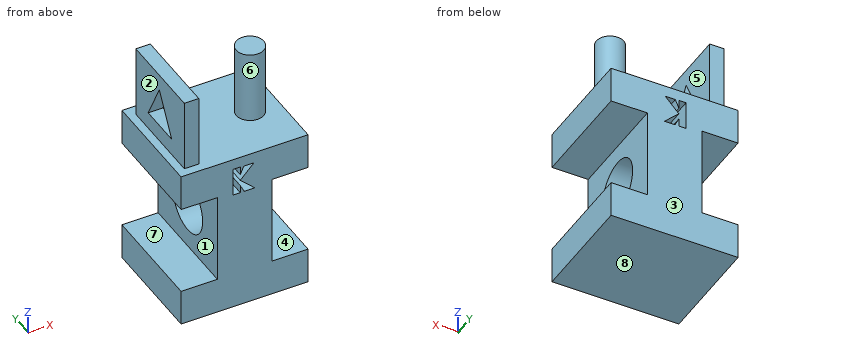
```python
from build123d import *

# Parameters (mm, degrees)
F1_DEPTH  = 76.2
F2_R      = 19.096035609
F3_DEPTH  = 47.498
F4_W      = 10.16
F4_H      = 62.4394440092
F5_DEPTH  = 50.8
F7_DEPTH  = 25.4
F9_DEPTH  = 96.52
F10_R     = 9.6573764136
F11_DEPTH = 50.8


# Not quite as in the source:
# - a feature names something its author has since deleted; it is built from what else it names


with BuildPart() as f1:
    # F0 (on Front) → F1 (new body)
    with BuildSketch(Plane.XZ):
        Polygon((-43.9144560635, -19.0287967878), (-43.9144560635, -44.4287967878), (44.9855439365, -44.4287967878), (44.9855439365, -19.0287967878), (19.5855439365, -19.0287967878), (19.5855439365, 44.4712032122), (44.9855439365, 44.4712032122), (44.9855439365, 69.8712032122), (-43.9144560635, 69.8712032122), (-43.9144560635, 44.4712032122), (-18.5144560635, 44.4712032122), (-18.5144560635, -19.0287967878), align=None)
    extrude(amount=F1_DEPTH)

    # F2 (on face) → F3 (cut)
    with BuildSketch(Plane.YZ.offset(19.5855439365)):
        with Locations((-38.1, 12.7212032122)):
            Circle(F2_R)
    extrude(amount=-F3_DEPTH, mode=Mode.SUBTRACT)

    # F4 (on face) → F5 (join)
    with BuildSketch(Plane.XY.offset(69.8712032122)):
        with Locations((-33.1311938035, -38.6642131489)):
            Rectangle(F4_W, F4_H)
    extrude(amount=F5_DEPTH)

    # F6 (on face) → F7 (cut)
    with BuildSketch(Plane(origin=(-38.2111938035, 0, 0), x_dir=(0, -1, 0), z_dir=(-1, 0, 0))):
        Polygon((53.6283701658, 81.7187428474), (37.7003215253, 109.3182116747), (23.2826862484, 81.7187428474), align=None)
    extrude(amount=-F7_DEPTH, mode=Mode.SUBTRACT)

    # F8 (on face) → F9 (cut)
    with BuildSketch(Plane(origin=(0, 0, 0), x_dir=(-1, 0, 0), z_dir=(0, 1, 0))):
        Polygon((7.511020638, 42.3752516508), (7.511020638, 62.378142029), (2.4668793194, 62.378142029), (2.4668793194, 56.307456918), (0, 62.0944574475), (-7.0838662127, 62.0944574475), (2.4668793194, 51.9569911986), (-7.7034849674, 42.3752516508), (-0.3085337383, 42.3752516508), (2.4668793194, 47.8559471667), (2.4668793194, 42.3752516508), align=None)
    extrude(amount=-F9_DEPTH, mode=Mode.SUBTRACT)

    # F10 (on face) → F11 (join)
    with BuildSketch(Plane.XY.offset(69.8712032122)):
        with Locations((25.0358451158, -38.1)):
            Circle(F10_R)
    extrude(amount=F11_DEPTH)


solid = f1.part
```
Check sheet for the modelled part. Datum: model origin and axes. Units: mm. Face numbers are marked on the shaded views. A direction names the side the tool comes from. Give positions to 0.01 mm unless a question says otherwise; leave off trailing zeros. Order: outer loops, then holes, each group sorted by start corner. A loop starts at its lowest first (then second) coordinate and runs counter-clockwise, first axis right, second up. Notation, with made-up numbers: (60.25, 47) -> (112.25, 47) arc R19 ccw to (112.25, 67) -> close; hole circle Ø6 at (-25.5, 71.25). An arc over 180 degrees is marked (long way). Use CSV: the item, a comma, the result in double quotes. Start each with the question number.
1) Sectioned sample at B-B, the plane y = -12. Record the boundary of the cut face in (x, z), plus the area to 3 significant figures.
2) Set-up check for the marked faces 1, 2, 3, 4 and 5: record each of +Z, -Z, +X, -X, +Y, -Y from which the full face is reachable in a straight line by a thin tool's end or side.
3) Material ranges on line 1 (Z direction, x = -3, y = -38.1); line 2 (Z direction, x = 10.5, y = -38.1); line 3 (Z direction, x = -21.5, y = -44), recorded low to high. Write a range as from..to.
4) Sectioned sample at C-C, the plane z = 50. Record the boundary of the cut face in (x, y), plus the area to 3 significant figures.
5) Mould release check, pull along Z, two halves, no side actions. Record for the marked faces 6, 7 and 8: released by +Z, released by -Z, zero draft, split by the parting line, or undercut.
6) Go/stop test with flat-tipped pins: P1, Ø3, axis at y = -26, z = 82, coming from the -X side; P2, Ø8, axis at y = -44, z = 36, coming from the +X side; P3, Ø11, axis at x = -31, z = 96, coming from the +Y side; P4, Ø23, axis at y = -38.1, z = 12.72, coming from the -X side. Record where each tip stops, or that it passes through.
7) Sectioned sample at A-A, the plane x = -32.5. Record the boundary of the cut face in (y, z).
8) Sectioned sample at D-D, the plane x = 3. Record the boundary of the cut face in (y, z).
Recorded:
1,outline,"(-43.91, -44.43) -> (44.99, -44.43) -> (44.99, -19.03) -> (19.59, -19.03) -> (19.59, 44.47) -> (44.99, 44.47) -> (44.99, 69.87) -> (-28.05, 69.87) -> (-28.05, 120.67) -> (-38.21, 120.67) -> (-38.21, 69.87) -> (-43.91, 69.87) -> (-43.91, 44.47) -> (-18.51, 44.47) -> (-18.51, -19.03) -> (-43.91, -19.03) -> close; hole (-7.51, 42.38) -> (-2.47, 42.38) -> (-2.47, 47.86) -> (0.31, 42.38) -> (7.7, 42.38) -> (-2.47, 51.96) -> (7.08, 62.09) -> (0, 62.09) -> (-2.47, 56.31) -> (-2.47, 62.38) -> (-7.51, 62.38) -> close"
1,area,"7,270 mm2"
2,face 1,"-X, +Y, -Y"
2,face 2,"+Z, -X, +Y, -Y"
2,face 3,"+Z, -Z, +X, -X, +Y"
2,face 4,"+X, +Y, -Y"
2,face 5,"+Z, +Y, -Y"
3,line 1,"-44.43..-6.37, 31.82..42.38, 62.38..69.87"
3,line 2,"-44.43..-6.37, 31.82..69.87"
3,line 3,"-44.43..-19.03, 44.47..69.87"
4,outline,"(-43.91, -76.2) -> (-7.51, -76.2) -> (-7.51, 0) -> (-43.91, 0) -> close; (-0.39, -76.2) -> (44.99, -76.2) -> (44.99, 0) -> (-0.39, 0) -> close"
4,area,"6,230 mm2"
5,face 6,"zero draft"
5,face 7,"undercut"
5,face 8,"released by -Z"
6,P1,"x = -38.21"
6,P2,"x = 19.59"
6,P3,"y = -7.44"
6,P4,"through"
7,outline,"(-76.2, -44.43) -> (0, -44.43) -> (0, -19.03) -> (-76.2, -19.03) -> close; (-76.2, 44.47) -> (0, 44.47) -> (0, 69.87) -> (-7.44, 69.87) -> (-7.44, 120.67) -> (-69.88, 120.67) -> (-69.88, 69.87) -> (-76.2, 69.87) -> close; hole (-53.63, 81.72) -> (-23.28, 81.72) -> (-37.7, 109.32) -> close"
8,outline,"(-76.2, -44.43) -> (0, -44.43) -> (0, 42.38) -> (-76.2, 42.38) -> close; (-76.2, 46.81) -> (0, 46.81) -> (0, 57.76) -> (-76.2, 57.76) -> close; (-76.2, 62.09) -> (0, 62.09) -> (0, 69.87) -> (-76.2, 69.87) -> close; hole circle Ø38.19 at (-38.1, 12.72)"
